```python
from build123d import *

# Parameters (mm, degrees)
SKETCH3_R            = 1.75
BOSS_EXTRUDE1_DEPTH  = 6
SKETCH4_W            = 10
SKETCH4_H            = 2.5
CUT_EXTRUDE1_DEPTH   = 10
CUT_REVOLVE1_ANGLE   = 180
CUT_EXTRUDE2_DEPTH   = 5
SKETCH10_R           = 0.5
CUT_EXTRUDE3_DEPTH   = 40
MIRROR6_COPY_1_ANGLE = 180
MIRROR6_COPY_2_DEPTH = 5
CUT_EXTRUDE4_DEPTH   = 6


with BuildPart() as part:
    # Sketch3 → Boss-Extrude1 (new body)
    with BuildSketch(Plane(origin=(0, 0, 0), x_dir=(1, 0, 0), z_dir=(0, 1, 0))):
        with BuildLine():
            Line((-23.265306122, 15.612244898), (16.734693878, 15.612244898))
            Line((16.734693878, 15.612244898), (21.734693878, 15.612244898))
            ThreePointArc((21.734693878, 15.612244898), (25.270227783, 14.147778804), (26.734693878, 10.612244898))
            Line((26.734693878, 10.612244898), (26.734693878, 6.112244898))
            ThreePointArc((26.734693878, 6.112244898), (26.588247268, 5.758691507), (26.234693878, 5.612244898))
            Line((26.234693878, 5.612244898), (16.734693878, 5.612244898))
            Line((16.734693878, 5.612244898), (16.734693878, 3.112244898))
            ThreePointArc((16.734693878, 3.112244898), (13.073528642, -5.726589867), (4.234693878, -9.387755102))
            Line((4.234693878, -9.387755102), (-10.765306122, -9.387755102))
            ThreePointArc((-10.765306122, -9.387755102), (-19.604140887, -5.726589867), (-23.265306122, 3.112244898))
            Line((-23.265306122, 3.112244898), (-23.265306122, 5.612244898))
            Line((-23.265306122, 5.612244898), (-32.765306122, 5.612244898))
            ThreePointArc((-32.765306122, 5.612244898), (-33.118859513, 5.758691507), (-33.265306122, 6.112244898))
            Line((-33.265306122, 6.112244898), (-33.265306122, 10.612244898))
            ThreePointArc((-33.265306122, 10.612244898), (-31.800840028, 14.147778804), (-28.265306122, 15.612244898))
            Line((-28.265306122, 15.612244898), (-23.265306122, 15.612244898))
        make_face()
        with Locations(Location((21.734693878, 10.612244898, 0), (0, 0, 270))):
            Circle(SKETCH3_R, mode=Mode.SUBTRACT)
        with Locations(Location((-28.265306122, 10.612244898, 0), (0, 0, 90))):
            Circle(SKETCH3_R, mode=Mode.SUBTRACT)
    extrude(amount=BOSS_EXTRUDE1_DEPTH)

    # Sketch4 → Cut-Extrude1 (cut)
    with BuildSketch(Plane(origin=(0, 0, -15.612244898), x_dir=(-1, 0, 0), z_dir=(0, 0, -1))):
        with Locations((28.265306122, 3)):
            Rectangle(SKETCH4_W, SKETCH4_H)
        with Locations((-21.734693878, 3)):
            Rectangle(SKETCH4_W, SKETCH4_H)
    extrude(amount=-CUT_EXTRUDE1_DEPTH, mode=Mode.SUBTRACT)

    # Sketch7 → Cut-Revolve1 (revolve, cut)
    with BuildSketch(Plane.XY.offset(-10.612244898)):
        Polygon((-33.265306122, 1.496669927), (-32.907482363, 1.496669927), (-32.015306122, 0.873334963), (-32.907482363, 0.25), (-33.265306122, 0.25), align=None)
    cut_revolve1 = revolve(axis=Axis((-28.265306122, 1.746669927, -10.612244898), (0, -1, 0)), revolution_arc=CUT_REVOLVE1_ANGLE, mode=Mode.SUBTRACT)

    # Sketch9 → Cut-Extrude2 (cut)
    with BuildSketch(Plane.XY.offset(-5.612244898)):
        Polygon((-23.623129882, 0.253330073), (-24.515306122, 0.876665037), (-23.623129882, 1.5), (-23.265306122, 1.5), (-23.265306122, 0.253330073), align=None)
    cut_extrude2 = extrude(amount=-CUT_EXTRUDE2_DEPTH, mode=Mode.SUBTRACT)

    # Sketch10 → Cut-Extrude3 (cut)
    with BuildSketch(Plane.ZY.offset(23.265306122)):
        with Locations((6.262755102, 0.875)):
            Circle(SKETCH10_R)
    cut_extrude3 = extrude(amount=-CUT_EXTRUDE3_DEPTH, mode=Mode.SUBTRACT)

    # Mirror5: Cut-Revolve1, Cut-Extrude2 across plane
    add(cut_revolve1.mirror(Plane.ZY.offset(3.265306122)), mode=Mode.SUBTRACT)
    add(cut_extrude2.mirror(Plane.ZY.offset(3.265306122)), mode=Mode.SUBTRACT)

    # Mirror6: Cut-Revolve1, Cut-Extrude2, Cut-Extrude3 across plane
    add(cut_revolve1.mirror(Plane.ZX.offset(3)), mode=Mode.SUBTRACT)
    add(cut_extrude2.mirror(Plane.ZX.offset(3)), mode=Mode.SUBTRACT)
    add(cut_extrude3.mirror(Plane.ZX.offset(3)), mode=Mode.SUBTRACT)

    # Mirror6 copy 1 sketch → Mirror6 copy 1 (revolve, cut)
    with BuildSketch(Plane(origin=(-6.530612245, 6, -10.612244898), x_dir=(-1, 0, 0), z_dir=(0, 0, 1))):
        Polygon((-33.265306122, 1.496669927), (-32.907482363, 1.496669927), (-32.015306122, 0.873334963), (-32.907482363, 0.25), (-33.265306122, 0.25), align=None)
    revolve(axis=Axis((21.734693878, 4.253330073, -10.612244898), (0, 1, 0)), revolution_arc=MIRROR6_COPY_1_ANGLE, mode=Mode.SUBTRACT)

    # Mirror6 copy 2 sketch → Mirror6 copy 2 (cut)
    with BuildSketch(Plane(origin=(-6.530612245, 6, -5.612244898), x_dir=(-1, 0, 0), z_dir=(0, 0, 1))):
        Polygon((-23.623129882, 0.253330073), (-24.515306122, 0.876665037), (-23.623129882, 1.5), (-23.265306122, 1.5), (-23.265306122, 0.253330073), align=None)
    extrude(amount=-MIRROR6_COPY_2_DEPTH, mode=Mode.SUBTRACT)

    # Sketch11 → Cut-Extrude4 (cut)
    with BuildSketch(Plane.XZ):
        with BuildLine():
            Line((11.734693878, -15.612244898), (-18.265306122, -15.612244898))
            ThreePointArc((-18.265306122, -15.612244898), (-3.265306122, -0.612244898), (11.734693878, -15.612244898))
        make_face()
    extrude(amount=-CUT_EXTRUDE4_DEPTH, mode=Mode.SUBTRACT)


solid = part.part
```
The listing builds one solid part. Answer for the finished solid, in the listing's coordinates (mm). A direction names the side the tool comes from. Coordinates: 2 decimals unless noted, no trailing zeros. Loops run counter-clockwise (first coordinate to the right, second up) from the corner with the lowest first, then second, coordinate; pieces in that order, holes last. Notation, with made-up numbers: (-4.75, 18) -> (34.25, 18) arc R16 ccw to (34.25, 43) -> close; hole circle Ø5 at (42.5, 83). An arc over 180 degrees is marked (long way). Use one line per item in the form item = value. Start each with the question number.
Item 1: Consider L1, parallel to Y at x = 24.5, z = -9.75; L2, parallel to X at y = 5.25, z = -10.5; L3, parallel to X at y = 3.75, z = -13.25. Determine where each line is inside the solid, lowest interval first. Write a range as [from, to].
Item 2: Flat-ended cylindrical pins translate along their axes: pin 1 Ø4 at (x, z) = (-25.5, 4) entering from +Y; pin 2 Ø3 at (x, y) = (20.5, 4) entering from +Z; pin 3 Ø1.5 at (y, z) = (4.5, 0.5) entering from +X; pin 4 Ø2 at (y, z) = (3, -10.5) entering from -X. Find the tip coordinate at first contact, or state that the pin passes through.
Item 3: The part is cut by section A-A on z = -4.25. Determine the outline of the cut face in (x, y), then the cut area to 3 significant figures.
Item 4: The part is cut by section C-C on x = -13. Determine the outline of the cut face in (y, z) (3 decimals), then the cut area to 3 significant figures.
Item 5: The part is cut by section B-B on y = 3.5. Determine the outline of the cut face in (x, z), then the cut area to 3 significant figures.
Item 6: A tool of negligible diameter and unlimited length cuts with its end or side. For faces 3 (the face through (-24.77, 0.88, -14.19)), 4 (the face through (22, 1, -5.612)), 5 (the face through (19.6, 4.25, -10.7)), 6 (the face through (16, 3, -15.612)), 7 (the face through (-33, 5, -10.612)), from which of +Z, -Z, +X, -X, +Y, -Y can it reach the whole face along a straight path? Write none if from no direction.
Item 7: The part is cut by section D-D on x = 19. Count the separate pieces of the cut face and the enclosed holes in it, then the cut area to 3 significant figures.
Item 8: The mould has two halves that part along Y. Classify faces 1 (the face through (-28.35, 0.97, -14.5)), 2 (the face through (-26.713, 0.863, -11.42)): released by +Y, released by -Y, zero draft, split by the parting line, or undercut.
Answer key:
q1.L1 = [0, 1.75], [4.25, 6]
q1.L2 = [-33.27, -30.01], [-26.52, -24.33], [-23.27, -17.37], [10.84, 16.73], [17.8, 19.99], [23.48, 26.73]
q1.L3 = [-23.27, -18.08], [11.55, 16.73]
q2.pin_1 = through
q2.pin_2 = -5.61
q2.pin_3 = 16.4
q2.pin_4 = -23.27
q3.outline = (-23.27, 0) -> (-13.06, 0) -> (-13.06, 6) -> (-23.27, 6) -> close; (6.53, 0) -> (16.73, 0) -> (16.73, 6) -> (6.53, 6) -> close
q3.area = 122 mm2
q4.outline = (0, -4.2) -> (6, -4.2) -> (6, 9.186) -> (0, 9.186) -> close; hole circle Ø1 at (0.875, 6.263); hole circle Ø1 at (5.125, 6.263)
q4.area = 78.7 mm2
q5.outline = (-23.27, -15.61) -> (-18.27, -15.61) arc R15 cw to (11.73, -15.61) -> (16.73, -15.61) -> (16.73, -3.11) arc R12.5 ccw to (4.23, 9.39) -> (-10.77, 9.39) arc R12.5 ccw to (-23.27, -3.11) -> close
q5.area = 580 mm2
q6.face_3 = none
q6.face_4 = +Z, +X, +Y, -Y
q6.face_5 = +Z, -Z, +X
q6.face_6 = -Z, +X, -X, +Y, -Y
q6.face_7 = -Z, -X
q7.separate_pieces = 2
q7.enclosed_holes = 2
q7.area = 32.5 mm2
q8.face_1 = undercut
q8.face_2 = zero draft
